Build history of the part. All positions in model axes, mm. A direction names the side the tool comes from. Give positions to 0.01 mm unless a question says otherwise; leave off trailing zeros. Write each loop counter-clockwise with the first axis right and the second up, starting at its lowest first coordinate (ties: lowest second). Pieces come first, ordered by that corner, then holes.
from build123d import *

# Parameters (mm, degrees)
F0_W     = 4
F0_H     = 40
F1_DEPTH = 20
F2_R     = 2.5
F3_DEPTH = 5
F4_R     = 2.5
F5_DEPTH = 10
F7_DEPTH = 4


with BuildPart() as f1:
    # F0 (on Right) → F1 (new body)
    with BuildSketch(Plane.YZ):
        Polygon((27.6797143764, -5), (27.6797143764, 0), (8.3147976454, 0), align=None)
        Polygon((8.3147976454, 0), (27.6797143764, 0), (27.6797143764, 5), (-22.3202856236, 5), (-22.3202856236, 0), (-18.3202856236, 0), align=None)
        with Locations((-20.3202856236, -20)):
            Rectangle(F0_W, F0_H)
    extrude(amount=F1_DEPTH)

    # F2 (on face) → F3 (cut)
    with BuildSketch(Plane.XZ.offset(22.3202856236)):
        with Locations((10, -25)):
            Circle(F2_R)
    extrude(amount=-F3_DEPTH, mode=Mode.SUBTRACT)

    # F4 (on face) → F5 (cut)
    with BuildSketch(Plane(origin=(0, 0.5196748528, 2.0126920505), x_dir=(1, 0, 0), z_dir=(0, -0.25, -0.9682458366))):
        with Locations((10, -18.0507682019)):
            Circle(F4_R)
    extrude(amount=-F5_DEPTH, mode=Mode.SUBTRACT)

    # F6 (on face) → F7 (cut)
    with BuildSketch(Plane.XY.offset(5)):
        Polygon((12.5, 18.4903720111), (12.5, 21.377123357), (10, 22.82049903), (7.5, 21.377123357), (7.5, 18.4903720111), (10, 17.0469963381), align=None)
    extrude(amount=-F7_DEPTH, mode=Mode.SUBTRACT)


solid = f1.part
1. 3-axis set-ups, long thin cutter, end or side, ignore diameter. For faces 4 (the face through (11.268, 22.089, 3.028)), 5 (the face through (9.67, -20.35, -22.52)), 6 (the face through (7.64, 20.01, -3.02)): which of +Z, -Z, +X, -X, +Y, -Y reach the whole face in a straight line?
2. Drill centre lines: line 1 along Z through (x, y) = (10, -20.55); line 2 along Y through (x, z) = (4.25, -25); line 3 along Z through (x, y) = (1.5, -3). Where is each one in solid material? Low to high.
3. Drop flat-ended pins along their axis: pin 1 (10 mm diameter, centred on x = 8.5, z = -28.5, fed in from +Y); pin 2 (10 mm diameter, centred on x = 10.5, y = -11, fed in from -Z); pin 3 (3 mm diameter, centred on x = 9.5, y = 20, fed in from +Z). Give the stop position or say it passes through.
4. Mould opens along X. For faces 1 (the face through (10, 27.68, 0)), 2 (the face through (20, -7, 1)), 3 (the face through (12.5, 20, 3)) say: pulls with the +X half, pulls with the -X half, needs draft (parallel to the pull), parting line crosses it, or undercut.
5. Saw through at D-D on y = 3. Give the cut face in (x, z), plus the area to 3 significant figures.
6. Saw through at B-B on x = 14.25. Give the cut face in (y, z), plus the area to 3 significant figures.
7. Saw through at A-A on z = -25. Give the cut face in (x, y), plus the area to 3 significant figures.
8. Saw through at C-C on z = -18. Give the cut face in (x, y), plus the area to 3 significant figures.
Outcome:
1. face 4: +Z
1. face 5: +Y, -Y
1. face 6: -Z, +X, -X
2. line 1: z = -40 to -27.5, -22.5 to 5
2. line 2: y = -22.32 to -18.32
2. line 3: z = 0 to 5
3. pin 1: stops at y = -18.32
3. pin 2: stops at z = 0
3. pin 3: stops at z = 1
4. face 1: needs draft
4. face 2: pulls with the +X half
4. face 3: undercut
5. outline: (0, 0) - (20, 0) - (20, 5) - (0, 5) - close
5. area: 100 mm2
6. outline: (-22.32, -40) - (-18.32, -40) - (-18.32, 0) - (8.31, 0) - (27.68, -5) - (27.68, 5) - (-22.32, 5) - close
6. area: 458 mm2
7. outline: (0, -22.32) - (7.5, -22.32) - (7.5, -18.32) - (0, -18.32) - close; (12.5, -22.32) - (20, -22.32) - (20, -18.32) - (12.5, -18.32) - close
7. area: 60.0 mm2
8. outline: (0, -22.32) - (20, -22.32) - (20, -18.32) - (0, -18.32) - close
8. area: 80.0 mm2
